Drawing for the job (mm, zero at the part's lowest x, y, z). A direction names the side the tool comes from. Coordinates: 2 decimals unless noted, no trailing zeros. Write each loop counter-clockwise with the first axis right and the second up, starting at its lowest first coordinate (ties: lowest second). Pieces come first, ordered by that corner, then holes. Notation, with made-up numbers: M 30.25,84 L 67.25,84 A32 cw 67.25,113 Z; hole C 12,-37 d5. An arc over 180 degrees is marked long. Use a Markdown table: item, result. Add a question column.
Q1. Slice it at D-D on y = 1. Write the cut outline in (x, z), then the cut area to 3 significant figures.
Q2. Slice it at C-C on z = 16.5. Write the cut outline in (x, y) (1 decimal).
Q3. Slice it at A-A on x = 14. Write the cut outline in (y, z), then the cut area to 3 significant figures.
Q4. Pin check, flat tips, straight feed: pin 1 Ø1 at (x, z) = (12, 32) entering from -Y; pin 2 Ø2 at (y, z) = (1.5, 34) entering from +X (1 decimal); pin 3 Ø2.5 at (y, z) = (2, 42.5) entering from +X; pin 4 Ø4 at (y, z) = (2.5, 41) entering from -X. Stop position of each tip, or through.
Q5. Wall check: L1, parallel to X at y = 6.25, z = 24; L2, parallel to X at y = 1.2, z = 24; L3, parallel to Z at x = 13.75, y = 6.5. Give the ranges that are in metal, low to high. Write a range as from..to.
Q6. Mould opens along X. For the marked faces 5, 6 and 7 say: released by +X, released by -X, zero draft, split by the parting line, or undercut.
Q7. Tool access for the marked faces 1, 2, 3 and 4: list every direction of +Z, -Z, +X, -X, +Y, -Y with a clear straight run to the whole face (end or side of a thin tool).
Q8. Slice it at B-B on y = 3.5. Write the cut outline in (x, z), then the cut area to 3 significant figures.
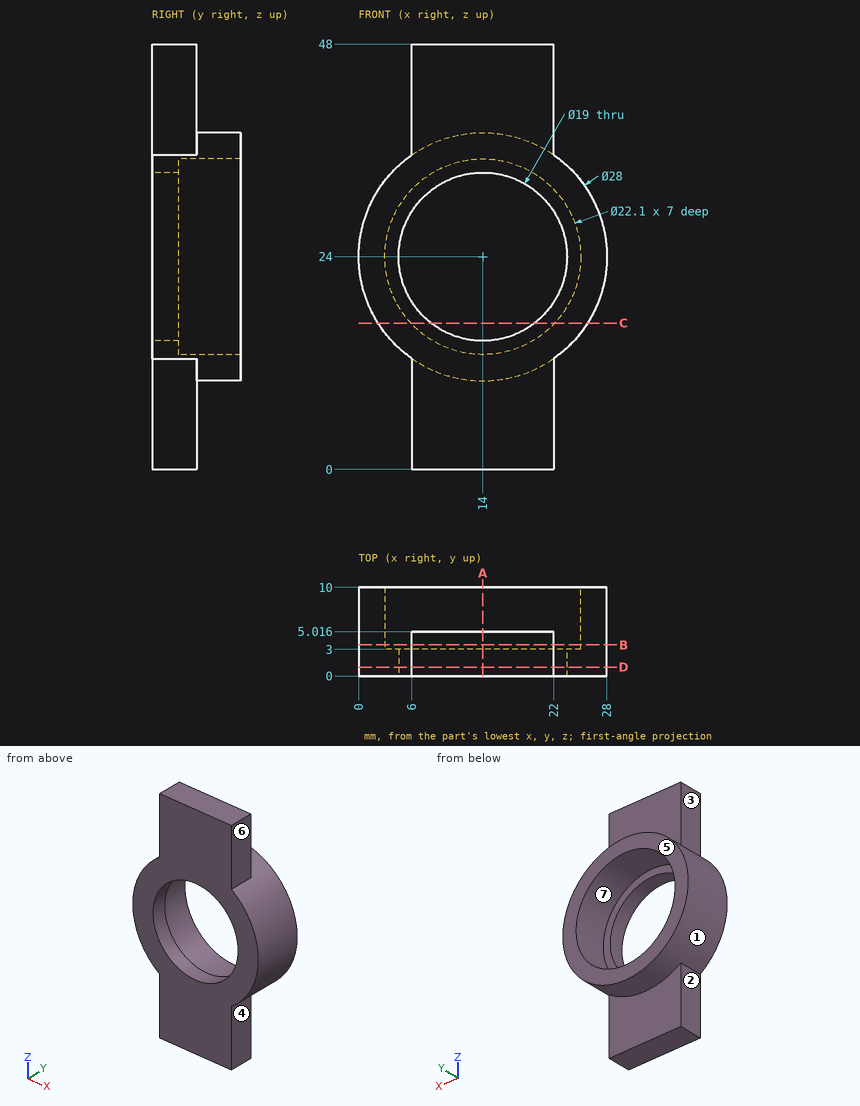
Recorded:
| question | item | result |
|---|---|---|
| 1 | outline | M 6,0 L 22,0 L 22,12.51 A14 ccw 22,35.49 L 22,48 L 6,48 L 6,35.49 A14 ccw 6,12.51 Z; hole C 14,24 d19 |
| 1 | area | 678 mm² |
| 2 | outline | M 2.2,0 L 8.2,0 L 8.2,3 L 5.9,3 L 5.9,10 L 2.2,10 Z; M 19.8,0 L 25.8,0 L 25.8,10 L 22.1,10 L 22.1,3 L 19.8,3 Z |
| 3 | outline | M 0,0 L 5.02,0 L 5.02,10 L 10,10 L 10,12.95 L 3,12.95 L 3,14.5 L 0,14.5 Z; M 0,33.5 L 3,33.5 L 3,35.05 L 10,35.05 L 10,38 L 5.02,38 L 5.02,48 L 0,48 Z |
| 3 | area | 169 mm² |
| 4 | pin 1 | through |
| 4 | pin 2 | x = 24.7 |
| 4 | pin 3 | x = 22 |
| 4 | pin 4 | x = 6 |
| 5 | L1 | 0..2.95, 25.05..28 |
| 5 | L2 | 0..4.5, 23.5..28 |
| 5 | L3 | 10..12.95, 35.05..38 |
| 6 | face 5 | zero draft |
| 6 | face 6 | released by +X |
| 6 | face 7 | undercut |
| 7 | face 1 | +Y |
| 7 | face 2 | -Z, -X, +Y, -Y |
| 7 | face 3 | +Z, -X, +Y, -Y |
| 7 | face 4 | -Z, +X, +Y, -Y |
| 8 | outline | M 6,0 L 22,0 L 22,12.51 A14 ccw 22,35.49 L 22,48 L 6,48 L 6,35.49 A14 ccw 6,12.51 Z; hole C 14,24 d22.1 |
| 8 | area | 578 mm² |
